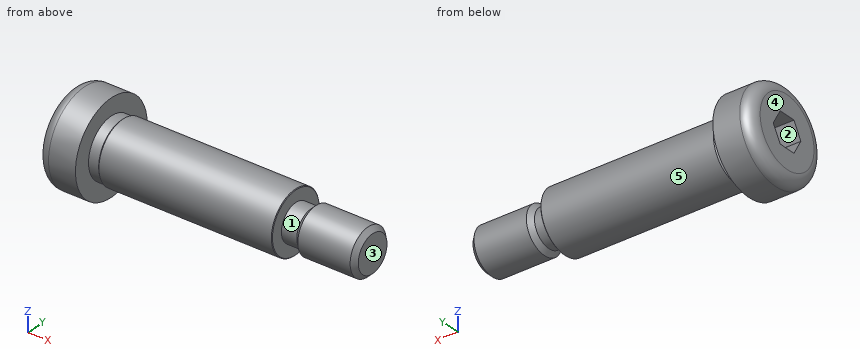
Autodesk Inventor part; units mm, degrees
ref_plane "YZ Plane" through (0, 0, 0) normal (1, 0, 0) x (0, 1, 0)
ref_plane "XZ Plane" through (0, 0, 0) normal (0, 1, 0) x (-1, 0, 0)
ref_plane "XY Plane" through (0, 0, 0) normal (0, 0, 1) x (1, 0, 0)
sketch "Sketch1" plane through (0, 0, 0) normal (0, 0, 1) x (1, 0, 0)
  line L0 (-1.0329, 0) -> (53.975, 0)
  line L1 (53.975, 0) -> (53.975, 4.7625)
  line L2 (53.975, 4.7625) -> (38.1, 4.7625)
  line L3 (38.1, 4.7625) -> (38.1, 6.3246)
  line L4 (38.1, 6.3246) -> (0, 6.3246)
  line L5 (0, 6.3246) -> (0, 9.525)
  line L6 (0, 9.525) -> (-7.9248, 9.525)
  line L7 (-7.9248, 9.525) -> (-7.9248, 3.6662)
  line L8 (-7.9248, 3.6662) -> (-3.1496, 3.6662)
  line L9 (-3.1496, 3.6662) -> (-1.0329, 0)
  line L10 (-20.3048, 0) -> (66.355, 0)
  line L11 (0, -1.905) -> (0, 11.43)
  line L12 (0, 6.0579) -> (2.0955, 6.0579)
  line L13 (2.0955, 6.0579) -> (2.3622, 6.3246)
  line L14 (38.1, 4.7625) -> (38.1, 3.8163)
  line L15 (38.1, 3.8163) -> (41.275, 3.8163)
  line L16 (41.275, 3.8163) -> (42.2212, 4.7625)
  line L17 (0, 6.0579) -> (0, 6.3246)
  dimension "d0" = 9.525
  dimension "d1" = 12.6492
  dimension "d2" = 19.05
  dimension "d3" = 7.3323
  dimension "d5" = 15.875
  dimension "d6" = 7.9248
  dimension "d7" = 4.7752
  dimension "d8" = 60
  dimension "d9" = 53.975
  dimension "d19" = 45
  dimension "d20" = 12.1158
  dimension "d21" = 7.6327
  dimension "d22" = 45
  dimension "d23" = 3.175
  dimension "d34" = 2.3622
revolve "Body" add sketch "Sketch1" angle 360 about axis through (-1.0329, 0, 0) along (1, 0, 0)
sketch "Sketch2" plane through (-7.9248, 0, 0) normal (-1, 0, 0) x (0, 0, 1)
  circle A0 centre (0, 0) radius 3.6662
  line L0 (0, 3.6662) -> (3.175, 1.8331)
  line L1 (3.175, 1.8331) -> (3.175, -1.8331)
  line L2 (3.175, -1.8331) -> (0, -3.6662)
  line L3 (0, -3.6662) -> (-3.175, -1.8331)
  line L4 (-3.175, -1.8331) -> (-3.175, 1.8331)
  line L5 (-3.175, 1.8331) -> (0, 3.6662)
extrude "Slot" add sketch "Sketch2" against normal up to next contours A0 L1 | L0 A0 | A0 L2 | L5 A0 | A0 L3 | L4 A0
fillet "Fillet1" radius 2.3622 1 edges at (-7.9248, -9.525, 0)
thread "Thread"
chamfer "Chamfer1" distance 0.9462 distance2 0.9461 1 edges at (53.975, -4.7625, 0) measured on face at (53.975, 0.1637, 0.4316)
chamfer "Chamfer2" distance 0.127 angle 45 1 edges at (38.1, -6.3246, 0) measured on face at (38.1, 5.6965, -0.8844)
revolve "Groove1" cut sketch "Sketch1" angle 360 about axis through (-1.0329, 0, 0) along (1, 0, 0) contours L11 L4 L13 L12
revolve "Groove2" cut sketch "Sketch1" angle 360 about axis through (-1.0329, 0, 0) along (1, 0, 0) contours L16 L15 L14 L2
equation "\"d0\" = NND"
equation "\"d1\" = BDM"
equation "\"d2\" = KOD"
equation "\"d3\" = 1.1547 * SW"
equation "\"d5\" = GEL"
equation "\"d6\" = KOH"
equation "\"d7\" = INTI + LOTI"
equation "\"d8\" = 0.5 * ANG"
equation "\"d9\" = NLG"
equation "\"d19\" = FAWI4"
equation "\"d20\" = BDMM"
equation "\"d21\" = GD1"
equation "\"d22\" = FAWI2"
equation "\"d23\" = GAL"
equation "\"d34\" = GAL2"
equation "\"d13\" = RR"
equation "\"d25\" = GEL"
equation "\"d14\" = -0.5 * SPD + 0.5 * NND"
equation "\"d15\" = GUL"
equation "\"d32\" = -0.5 * NND + 0.5 * BDM"
equation "\"NND\" = 9.525"
equation "\"NLG\" = 53.975"
equation "\"GEL\" = 15.875"
equation "\"KOD\" = 19.05"
equation "\"KOH\" = 7.9248"
equation "\"INTI\" = 4.7752"
equation "\"GAL\" = 3.175"
equation "\"GUL\" = 0.94615"
equation "\"SPD\" = GD1"
equation "\"BDM\" = 12.6492"
equation "\"ANG\" = 120deg"
equation "\"FAWI2\" = 45deg"
equation "\"FAWI3\" = 45deg"
equation "\"FAWI4\" = 45deg"
equation "\"RR\" = 2.3622"
equation "\"SW\" = 6.35"
equation "\"BDMM\" = 12.1158"
equation "\"GAL2\" = RR"
equation "\"LOTI\" = 0"
equation "\"GD1\" = 7.6327"
equation "\"BOR\" = SW"
equation "\"SLG\" = 38.1"
equation "\"THREADDIA\" = 9.525"
equation "\"E0\" = 1.155 * SW"
equation "\"FAWI1\" = 45deg"
equation "\"TOA\" = 30deg"
equation "\"PHH\" = RR"
equation "\"HHPTC\" = 1.5875"
equation "\"GD0\" = 7.3914"
equation "\"KOH1\" = 6.6548"
equation "\"BDMN\" = 12.7"
properties part number "ANSI B18.3 - 0.500 x 1.5 ANSI B18.3" material "Steel, Mild"
The model under review builds one solid part; all positions refer to its coordinate system, in mm. Face numbers are marked on the shaded views. A direction names the side the tool comes from. Give positions to 0.01 mm unless a question says otherwise; leave off trailing zeros. Write each loop counter-clockwise with the first axis right and the second up, starting at its lowest first coordinate (ties: lowest second). Pieces come first, ordered by that corner, then holes.
1. For P1, Ø4, axis at x = 1.5, z = 7.5, coming from the +Y side; P2, Ø3, axis at x = 33, z = 1.5, coming from the -Y side; P3, Ø5, axis at y = 3, z = 1, coming from the -X side; P4, Ø8, axis at x = 22.5, y = 3, coming from the -Z side, all flat-tipped, find the tip position at first contact; note any pin that passes through.
2. Add section A-A, the plane x = 16. Write out the cut boundary in (y, z).
3. Add section B-B, the plane x = 46. Write out the cut boundary in (y, z) (1 decimal), plus the area to 3 significant figures.
4. Draft analysis for pull direction X (two halves, no side actions). For the marked faces 1, 2 and 3, state which applies: +X half, -X half, draft (parallel to the pull), parting line (faces both ways), or undercut.
5. Wall thickness on L1, parallel to X at y = -7, z = -1.25; L2, parallel to Z at x = 19, y = 0.25; L3, parallel to X at y = 2.75, z = -4.75: over which ranges is each line inside the solid? List them lowest first.
6. Tool access review of the marked faces 4 and 5: name each direction out of +Z, -Z, +X, -X, +Y, -Y from which nothing blocks a thin tool from reaching the whole face with its end or side.
Worked answers:
1. P1: stops at y = 7.25
1. P2: stops at y = -6.32
1. P3: stops at x = -7.92
1. P4: stops at z = -6.32
2. outline: circle Ø12.65 at (0, 0)
3. outline: circle Ø9.5 at (0, 0)
3. area: 71.3 mm2
4. face 1: undercut
4. face 2: draft
4. face 3: +X half
5. L1: x = -7.92 to 0
5. L2: z = -6.32 to 6.32
5. L3: x = -7.92 to 38.1
6. face 4: +Z, -Z, -X, +Y, -Y
6. face 5: +X
